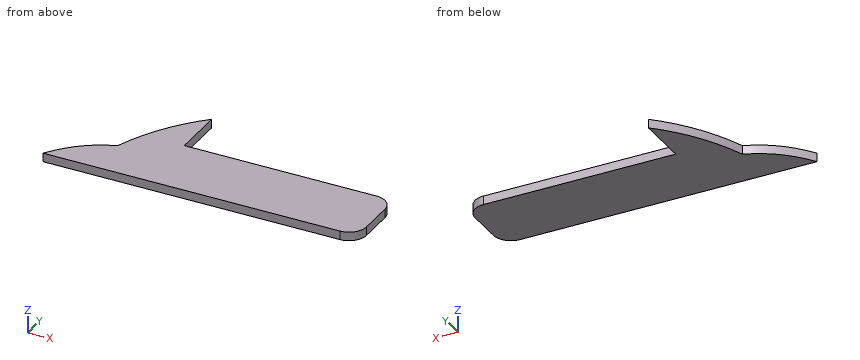
from build123d import *

# Parameters (mm, degrees)
BOSS_EXTRUDE1_DEPTH = 12.7


with BuildPart() as part:
    # Sketch2 → Boss-Extrude1 (new body)
    with BuildSketch(Plane.XY):
        with BuildLine():
            Line((0, 0), (431.8, 0))
            ThreePointArc((431.8, 0), (449.760512242, 7.439487758), (457.2, 25.4))
            Line((457.2, 25.4), (457.2, 76.2))
            ThreePointArc((457.2, 76.2), (449.760512242, 94.160512242), (431.8, 101.6))
            Line((431.8, 101.6), (152.4, 101.6))
            Line((152.4, 101.6), (152.4, 177.8))
            add(Edge.make_bspline(
                [(76.2, 61.401256844), (101.247409755, 131.199229676), (152.4, 177.8)],
                knots=[0, 0, 0, 0.857766608, 0.857766608, 0.857766608], degree=2))
            add(Edge.make_bspline(
                [(0, 0), (29.783016718, 46.127848409), (76.2, 61.401256844)],
                knots=[0, 0, 0, 0.939645984, 0.939645984, 0.939645984], degree=2))
        make_face()
    extrude(amount=BOSS_EXTRUDE1_DEPTH)


solid = part.part
The listing builds one solid part. Answer for the finished solid, in the listing's coordinates (mm). Coordinates: 2 decimals unless noted, no trailing zeros. Loops run counter-clockwise (first coordinate to the right, second up) from the corner with the lowest first, then second, coordinate; pieces in that order, holes last. Notation, with made-up numbers: (-12.5, 72) -> (40.5, 72) arc R28 cw to (40.5, 103) -> close; hole circle Ø10 at (59.5, 39.5). An arc over 180 degrees is marked (long way). Answer in a Markdown table with one row per item. Add a question column.
1. Consider line 1 (Y direction, x = 197, z = 9); line 2 (X direction, y = 123.5, z = 3.5); line 3 (X direction, y = 36, z = 6.25). Determine where each line is inside the solid, lowest interval first. Write a range as [from, to].
2. The part is cut by section A-A, the plane x = 345. Write down the section's boundary in (y, z), then the cut area to 3 significant figures.
3. Flat-ended cylindrical pins translate along their axes: P1, Ø4, axis at x = 234.5, z = 6, coming from the +Y side; P2, Ø10, axis at x = 102.5, y = 58.5, coming from the -Z side; P3, Ø3, axis at y = 144.5, z = 6.5, coming from the +X side; P4, Ø3, axis at y = 87.5, z = 8.5, coming from the -X side. Find the tip coordinate at first contact, or state that the pin passes through.
Answer below:
| question | item | result |
|---|---|---|
| 1 | line 1 | [0, 101.6] |
| 1 | line 2 | [106.54, 152.4] |
| 1 | line 3 | [31.03, 457.2] |
| 2 | outline | (0, 0) -> (101.6, 0) -> (101.6, 12.7) -> (0, 12.7) -> close |
| 2 | area | 1,290 mm2 |
| 3 | P1 | y = 101.6 |
| 3 | P2 | z = 0 |
| 3 | P3 | x = 152.4 |
| 3 | P4 | x = 86.16 |
